from build123d import *

# Parameters (mm, degrees)
F0_W     = 38.1
F0_H     = 38.1
F0_R     = 9.525
F1_DEPTH = 6.35
F2_SIZE  = 2.54
F3_SIZE  = 2.54


with BuildPart() as f1:
    # F0 (on Front) → F1 (new body)
    with BuildSketch(Plane.XZ):
        with Locations((19.05, 19.05)):
            Rectangle(F0_W, F0_H)
        with Locations((19.05, 19.05)):
            Circle(F0_R, mode=Mode.SUBTRACT)
        Polygon((19.05, 71.095568), (0, 38.1), (38.1, 38.1), align=None)
        Polygon((-32.995568, 19.05), (0, 0), (0, 38.1), align=None)
        Polygon((38.1, 38.1), (38.1, 0), (71.095568, 19.05), align=None)
        Polygon((38.1, 0), (0, 0), (19.05, -32.995568), align=None)
    extrude(amount=F1_DEPTH)

    # F2
    f2_edges = [f1.edges().sort_by_distance(p)[0] for p in [
        (9.525, -6.35, 54.597784),
        (-16.497784, -6.35, 28.575),
        (-16.497784, -6.35, 9.525),
        (9.525, -6.35, -16.497784),
        (28.575, -6.35, -16.497784),
        (54.597784, -6.35, 9.525),
        (54.597784, -6.35, 28.575),
        (28.575, -6.35, 54.597784),
    ]]
    chamfer(f2_edges, length=F2_SIZE)

    # F3
    f3_edges = [f1.edges().sort_by_distance(p)[0] for p in [
        (9.525, 0, -16.497784),
        (28.575, 0, -16.497784),
        (54.597784, 0, 9.525),
        (54.597784, 0, 28.575),
        (28.575, 0, 54.597784),
        (9.525, 0, 54.597784),
        (-16.497784, 0, 28.575),
        (-16.497784, 0, 9.525),
    ]]
    chamfer(f3_edges, length=F3_SIZE)


solid = f1.part
For this review, take the finished solid that the model builds, in its own axes (mm). Round coordinates to 2 decimals unless told otherwise and drop trailing zeros. Loops run counter-clockwise (first coordinate to the right, second up) from the corner with the lowest first, then second, coordinate; pieces in that order, holes last. Notation, with made-up numbers: (14.25, 80) - (56.25, 80) arc R29 ccw to (56.25, 118) - close; hole circle Ø5 at (38.5, -38). An arc over 180 degrees is marked (long way). Put each result on its own line as item: value. Start each with the question number.
1. Consider section D-D on z = 7. State the section outline as (x, y) points.
2. Mouldability with a two-part tool opening along Z and no side actions: class faces 1 (the cylindrical face through (16.99, -3.13, 9.75)), 2 (the flat face through (27.8, -1.29, 53.44)), 3 (the flat face through (12, -6.35, 26)) as +Z half, -Z half, draft (parallel to the pull), parting line (faces both ways), or undercut.
3. For probe 1 along X at (y, z) = (-0.25, 18); probe 2 along X at (y, z) = (-3, 16); probe 3 along X at (y, z) = (-2, 60), list the stretches that pass through material, from the lowest coordinate up. Write a range as [from, to].
4. Insertion check: P1, Ø2, axis at y = -4.5, z = 44, coming from the +X side; P2, Ø1, axis at y = -3.5, z = -17.5, coming from the +X side; P3, Ø1, axis at y = -1.5, z = -18.5, coming from the -X side. Each pin has a flat end and moves straight along its axis. Give the tip position at first contact, or say it passes through.
5. Consider section B-B on x = 17.5. State the section outline as (y, z) points.
6. Consider section A-A on y = -1.5. State the section outline as (x, z) points (3 decimals).
7. Consider section C-C on x = -3. State the section outline as (y, z) points (3 decimals), plus the area to 3 significant figures.
Result sheet:
1. outline: (-12.12, -3.81) - (-7.04, -6.35) - (45.14, -6.35) - (50.22, -3.81) - (50.22, -2.54) - (45.14, 0) - (-7.04, 0) - (-12.12, -2.54) - close
2. face 1: undercut
2. face 2: +Z half
2. face 3: draft
3. probe 1: [-26.6, 9.58], [28.52, 64.7]
3. probe 2: [-27.71, 10.03], [28.07, 65.81]
3. probe 3: [13.27, 24.83]
4. P1: x = 35.11
4. P2: x = 28.29
4. P3: x = 11.24
5. outline: (-6.35, -25.23) - (-3.81, -30.31) - (-2.54, -30.31) - (0, -25.23) - (0, 9.65) - (-6.35, 9.65) - close; (-6.35, 28.45) - (0, 28.45) - (0, 63.33) - (-2.54, 68.41) - (-3.81, 68.41) - (-6.35, 63.33) - close
6. outline: (-30.916, 19.05) - (0.761, 0.761) - (19.05, -30.916) - (37.339, 0.761) - (69.016, 19.05) - (37.339, 37.339) - (19.05, 69.016) - (0.761, 37.339) - close; hole circle Ø19.05 at (19.05, 19.05)
7. outline: (-6.35, 4.665) - (-3.81, 1.732) - (-2.54, 1.732) - (0, 4.665) - (0, 33.435) - (-2.54, 36.368) - (-3.81, 36.368) - (-6.35, 33.435) - close
7. area: 205 mm^2
